Design review of the part built by this model. Coordinates are the model's own, in mm. Give positions to 0.01 mm unless a question says otherwise; leave off trailing zeros. Order: outer loops, then holes, each group sorted by start corner. A loop starts at its lowest first (then second) coordinate and runs counter-clockwise, first axis right, second up. Notation, with made-up numbers: (51.5, -25.5) -> (74.5, -25.5) arc R3 ccw to (74.5, -20.5) -> close; hole circle Ø1 at (46, 6.25). An arc over 180 degrees is marked (long way). Answer in a Markdown table with one row per item. Add a question column.
```python
from build123d import *

# Parameters (mm, degrees)
SKETCH1_W           = 101.6
SKETCH1_H           = 50.8
BOSS_EXTRUDE1_DEPTH = 9.525
CHAMFER1_SIZE       = 1.27
SKETCH2_R           = 3.175
CUT_EXTRUDE1_DEPTH  = 58.589283942


with BuildPart() as part:
    # Sketch1 → Boss-Extrude1 (new body)
    with BuildSketch(Plane(origin=(0, 0, 0), x_dir=(1, 0, 0), z_dir=(0, 1, 0))):
        Rectangle(SKETCH1_W, SKETCH1_H)
    extrude(amount=BOSS_EXTRUDE1_DEPTH)

    # Chamfer1
    chamfer1_edges = [part.edges().sort_by_distance(p)[0] for p in [
        (50.8, 9.525, 0),
        (0, 9.525, -25.4),
        (-50.8, 9.525, 0),
        (0, 0, -25.4),
        (50.8, 0, 0),
        (0, 0, 25.4),
        (-50.8, 0, 0),
        (-50.8, 4.7625, -25.4),
        (50.8, 4.7625, -25.4),
        (50.8, 4.7625, 25.4),
        (-50.8, 4.7625, 25.4),
        (0, 9.525, 25.4),
    ]]
    chamfer(chamfer1_edges, length=CHAMFER1_SIZE)

    # Sketch2 → Cut-Extrude1 (cut, through all)
    with BuildSketch(Plane(origin=(0, 9.525, 0), x_dir=(1, 0, 0), z_dir=(0, 1, 0))):
        with Locations(Location((-38.1, 19.05, 0), (0, 0, 270))):
            Circle(SKETCH2_R)
        with Locations(Location((-38.1, -19.05, 0), (0, 0, 270))):
            Circle(SKETCH2_R)
        with Locations(Location((38.1, -19.05, 0), (0, 0, 270))):
            Circle(SKETCH2_R)
        with Locations(Location((38.1, 19.05, 0), (0, 0, 270))):
            Circle(SKETCH2_R)
    extrude(amount=-CUT_EXTRUDE1_DEPTH, mode=Mode.SUBTRACT)


solid = part.part
```
1) Add section B-B, the plane x = -38.1. Write out the cut boundary in (y, z) (3 decimals).
2) Add section A-A, the plane z = 19.05. Write out the cut boundary in (x, y) (3 decimals).
3) For L1, parallel to X at y = 5.5, z = 19.05 (3 decimals); L2, parallel to Z at x = 39, y = 7; L3, parallel to X at y = 9.25, z = -19 (3 decimals), list the stretches that pass through material, from the lowest coordinate up.
4) Add section C-C, the plane y = 5.25. Write out the cut boundary in (x, z) (3 decimals).
5) Mouldability with a two-part tool opening along X and no side actions: class faces 1 (the face through (-50.8, 5, 0)), 2 (the face through (-1, 9.525, 0)), 3 (the face through (50.8, 5, 0)), 4 (the face through (-35.954, 4.829, 16.71)) as +X half, -X half, draft (parallel to the pull), parting line (faces both ways), or undercut.
Verdict:
| question | item | result |
|---|---|---|
| 1 | outline | (0, -24.13) -> (1.27, -25.4) -> (8.255, -25.4) -> (9.525, -24.13) -> (9.525, -22.225) -> (0, -22.225) -> close; (0, -15.875) -> (9.525, -15.875) -> (9.525, 15.875) -> (0, 15.875) -> close; (0, 22.225) -> (9.525, 22.225) -> (9.525, 24.13) -> (8.255, 25.4) -> (1.27, 25.4) -> (0, 24.13) -> close |
| 2 | outline | (-50.8, 1.27) -> (-49.53, 0) -> (-41.275, 0) -> (-41.275, 9.525) -> (-49.53, 9.525) -> (-50.8, 8.255) -> close; (-34.925, 0) -> (34.925, 0) -> (34.925, 9.525) -> (-34.925, 9.525) -> close; (41.275, 0) -> (49.53, 0) -> (50.8, 1.27) -> (50.8, 8.255) -> (49.53, 9.525) -> (41.275, 9.525) -> close |
| 3 | L1 | x = -50.8 to -41.275, -34.925 to 34.925, 41.275 to 50.8 |
| 3 | L2 | z = -25.4 to -22.09, -16.01 to 16.01, 22.09 to 25.4 |
| 3 | L3 | x = -49.805 to -41.275, -34.925 to 34.925, 41.275 to 49.805 |
| 4 | outline | (-50.8, -24.13) -> (-49.53, -25.4) -> (49.53, -25.4) -> (50.8, -24.13) -> (50.8, 24.13) -> (49.53, 25.4) -> (-49.53, 25.4) -> (-50.8, 24.13) -> close; hole circle Ø6.35 at (-38.1, -19.05); hole circle Ø6.35 at (-38.1, 19.05); hole circle Ø6.35 at (38.1, -19.05); hole circle Ø6.35 at (38.1, 19.05) |
| 5 | face 1 | -X half |
| 5 | face 2 | draft |
| 5 | face 3 | +X half |
| 5 | face 4 | undercut |
